Here's how the part is built. I have some questions about the finished solid (model axes, mm). A direction names the side the tool comes from. Round coordinates to 2 decimals unless told otherwise and drop trailing zeros. Loops run counter-clockwise (first coordinate to the right, second up) from the corner with the lowest first, then second, coordinate; pieces in that order, holes last. Notation, with made-up numbers: (12, 2.25) - (32, 2.25) arc R30 ccw to (32, 41.25) - close; hole circle Ø10 at (-3.5, -16). An arc over 180 degrees is marked (long way). Return JSON: item names as keys, results as strings. Group by question number.
```python
from build123d import *

# Parameters (mm, degrees)
BOSS_EXTRUDE1_DEPTH                               = 5
CBORE_FOR_M2_5_SOCKET_HEAD_CAP_SCREW1_D           = 2.9
CBORE_FOR_M2_5_SOCKET_HEAD_CAP_SCREW1_CBORE_D     = 5.5
CBORE_FOR_M2_5_SOCKET_HEAD_CAP_SCREW1_CBORE_DEPTH = 2.5
SKETCH6_W                                         = 113
SKETCH6_H                                         = 36
BOSS_EXTRUDE2_DEPTH                               = 5
BOSS_EXTRUDE3_DEPTH                               = 5
SKETCH8_R                                         = 9.75
CUT_EXTRUDE1_DEPTH                                = 5
M2_5_TAPPED_HOLE1_D                               = 2.05


with BuildPart() as part:
    # Sketch1 → Boss-Extrude1 (new body)
    with BuildSketch(Plane(origin=(0, 0, 0), x_dir=(0, 0, -1), z_dir=(1, 0, 0))):
        with BuildLine():
            Line((0, 18), (45, 18))
            Line((45, 18), (45, -18))
            Line((45, -18), (0, -18))
            ThreePointArc((0, -18), (-18, 0), (0, 18))
        make_face()
    extrude(amount=BOSS_EXTRUDE1_DEPTH)

    # CBORE for M2.5 Socket Head Cap Screw1 (through all)
    with Locations(Plane(origin=(5, 14, 0), x_dir=(0, 0, 1), z_dir=(1, 0, 0))):
        with Locations((0, 0), (-14, 14), (0, 28), (14, 14)):
            CounterBoreHole(CBORE_FOR_M2_5_SOCKET_HEAD_CAP_SCREW1_D / 2, CBORE_FOR_M2_5_SOCKET_HEAD_CAP_SCREW1_CBORE_D / 2, CBORE_FOR_M2_5_SOCKET_HEAD_CAP_SCREW1_CBORE_DEPTH)

    # Sketch6 → Boss-Extrude2 (add)
    with BuildSketch(Plane(origin=(0, 0, -45), x_dir=(-1, 0, 0), z_dir=(0, 0, -1))):
        with Locations((51.5, 0)):
            Rectangle(SKETCH6_W, SKETCH6_H)
    extrude(amount=BOSS_EXTRUDE2_DEPTH)

    # Sketch7 → Boss-Extrude3 (add)
    with BuildSketch(Plane.ZY.offset(108)):
        with BuildLine():
            Line((-50, -18), (0, -18))
            ThreePointArc((0, -18), (18, 0), (0, 18))
            Line((0, 18), (-50, 18))
            Line((-50, 18), (-50, -18))
        make_face()
    extrude(amount=-BOSS_EXTRUDE3_DEPTH)

    # Sketch8 → Cut-Extrude1 (cut)
    with BuildSketch(Plane.ZY.offset(108)):
        Circle(SKETCH8_R)
    extrude(amount=-CUT_EXTRUDE1_DEPTH, mode=Mode.SUBTRACT)

    # M2.5 Tapped Hole1 (through all)
    with Locations(Plane(origin=(0, 0, -50), x_dir=(-1, 0, 0), z_dir=(0, 0, -1))):
        with Locations((36.5, 10), (66.5, 10), (66.5, -10), (36.5, -10)):
            Hole(M2_5_TAPPED_HOLE1_D / 2)


solid = part.part
```
Q1. Imagine slicing it at A-A, the plane z = -14. List the corners of the cut face in (x, y) for me, and give its area (3 significant figures).
Q2. Imagine slicing it at D-D, the plane y = -14. List the corners of the cut face in (x, z) for me.
Q3. For faces 5 (the flat face through (-51, 0, -45)), 6 (the flat face through (-108, 0, -23)), 7 (the cylindrical face through (-105.535, 9.667, -1.269)), 8 (the flat face through (2.5, -12.8, 1.2)), which set-ups out of +Z, -Z, +X, -X, +Y, -Y let a thin tool reach every point of the face, with its end or its side?
Q4. Please list where these lines run through material, in increasing order: line 1 (Y direction, x = -66.5, z = -46.3) (3 decimals); line 2 (X direction, y = -9, z = 8); line 3 (Y direction, x = 3, z = 0).
Q5. Will these pins go through, and if not, where does the flat tip stop? pin 1 Ø1.5 at (x, y) = (-69.5, 1.5) entering from +Z; pin 2 Ø3.5 at (y, z) = (-14, 0) entering from +X; pin 3 Ø9 at (y, z) = (14, 0) entering from +X; pin 4 Ø1.6 at (y, z) = (0, 13.5) entering from +X.
Q6. Imagine slicing it at B-B, the plane y = 0. List the corners of the cut face in (x, z) for me.
Q7. If we mould it in two halves opening along Y, with no side actions, what happens to faces 1 (the flat face through (-51, 0, -50)), 2 (the cylindrical face through (2, 0, 18)), 3 (the cylindrical face through (3.768, -0.121, -16.747)), 4 (the flat face through (-51, 18, -47))? For each: +Y half, -Y half, draft (parallel to the pull), parting line (faces both ways), or undercut.
Q8. Imagine slicing it at C-C, the plane z = -33.5. List the corners of the cut face in (x, y) for me.
Output values:
{
 "1": {"outline": "(-108, -18) - (-103, -18) - (-103, 18) - (-108, 18) - close; (0, -18) - (5, -18) - (5, -2.75) - (2.5, -2.75) - (2.5, -1.45) - (0, -1.45) - close; (0, 1.45) - (2.5, 1.45) - (2.5, 2.75) - (5, 2.75) - (5, 18) - (0, 18) - close", "area": "339 mm^2"},
 "2": {"outline": "(-108, -50) - (5, -50) - (5, -2.75) - (2.5, -2.75) - (2.5, -1.45) - (0, -1.45) - (0, -45) - (-103, -45) - (-103, 11.31) - (-108, 11.31) - close; (0, 1.45) - (2.5, 1.45) - (2.5, 2.75) - (5, 2.75) - (5, 11.31) - (0, 11.31) - close"},
 "3": {"face 5": "+Z, +Y, -Y", "face 6": "+Z, -Z, -X, +Y, -Y", "face 7": "-X", "face 8": "+X"},
 "4": {"line 1": "y = -18 to -11.025, -8.975 to 8.975, 11.025 to 18", "line 2": "x = -108 to -103, 0 to 5", "line 3": "y = -18 to -16.75, -11.25 to 11.25, 16.75 to 18"},
 "5": {"pin 1": "stops at z = -45", "pin 2": "stops at x = 2.5", "pin 3": "stops at x = 5", "pin 4": "stops at x = -103"},
 "6": {"outline": "(-108, -50) - (5, -50) - (5, -16.75) - (2.5, -16.75) - (2.5, -15.45) - (0, -15.45) - (0, -45) - (-103, -45) - (-103, -9.75) - (-108, -9.75) - close; (-108, 9.75) - (-103, 9.75) - (-103, 18) - (-108, 18) - close; (0, -12.55) - (2.5, -12.55) - (2.5, -11.25) - (5, -11.25) - (5, 11.25) - (2.5, 11.25) - (2.5, 12.55) - (0, 12.55) - close; (0, 15.45) - (2.5, 15.45) - (2.5, 16.75) - (5, 16.75) - (5, 18) - (0, 18) - close"},
 "7": {"face 1": "draft", "face 2": "parting line", "face 3": "undercut", "face 4": "+Y half"},
 "8": {"outline": "(-108, -18) - (-103, -18) - (-103, 18) - (-108, 18) - close; (0, -18) - (5, -18) - (5, 18) - (0, 18) - close"}
}
